Part print with two shaded views. Sizes in mm from the minimum x, y, z corner. A direction names the side the tool comes from. Coordinates: 2 decimals unless noted, no trailing zeros. Loops run counter-clockwise (first coordinate to the right, second up) from the corner with the lowest first, then second, coordinate; pieces in that order, holes last.
Item 1: Cut at C-C (y = 7). List the corners of the cut face in (x, z).
Item 2: Cut at B-B (z = 50). List the corners of the cut face in (x, y), and give its area (3 significant figures).
Item 3: Drill centre lines: line 1 along Z through (x, y) = (31, 47); line 2 along Y through (x, z) = (15, 33); line 3 along Z through (x, y) = (22.5, 21). Where is each one in solid material? Low to high.
Item 4: 3-axis set-ups, long thin cutter, end or side, ignore diameter. For the marked faces 1, 2 and 3: which of +Z, -Z, +X, -X, +Y, -Y reach the whole face in a straight line?
Item 5: Mould opens along X. For the marked faces 4, 5 and 6 say: released by +X, released by -X, zero draft, split by the parting line, or undercut.
Item 6: Flat gauge pins, fed straight in: pin 1 (14 mm diameter, centred on x = 24, z = 4, fed in from -Y); pin 2 (2 mm diameter, centred on x = 20.5, y = 37, fed in from +Z); pin 3 (12 mm diameter, centred on y = 38.5, z = 37.5, fed in from +X); pin 4 (2.5 mm diameter, centred on y = 3.5, z = 9.5, fed in from -X) (1 decimal). Where does each tip first touch, or does it go through?
Item 7: Cut at A-A (x = 31.75). List the corners of the cut face in (y, z), and give its area (3 significant figures).
Item 8: Cut at D-D (y = 15). List the corners of the cut face in (x, z).
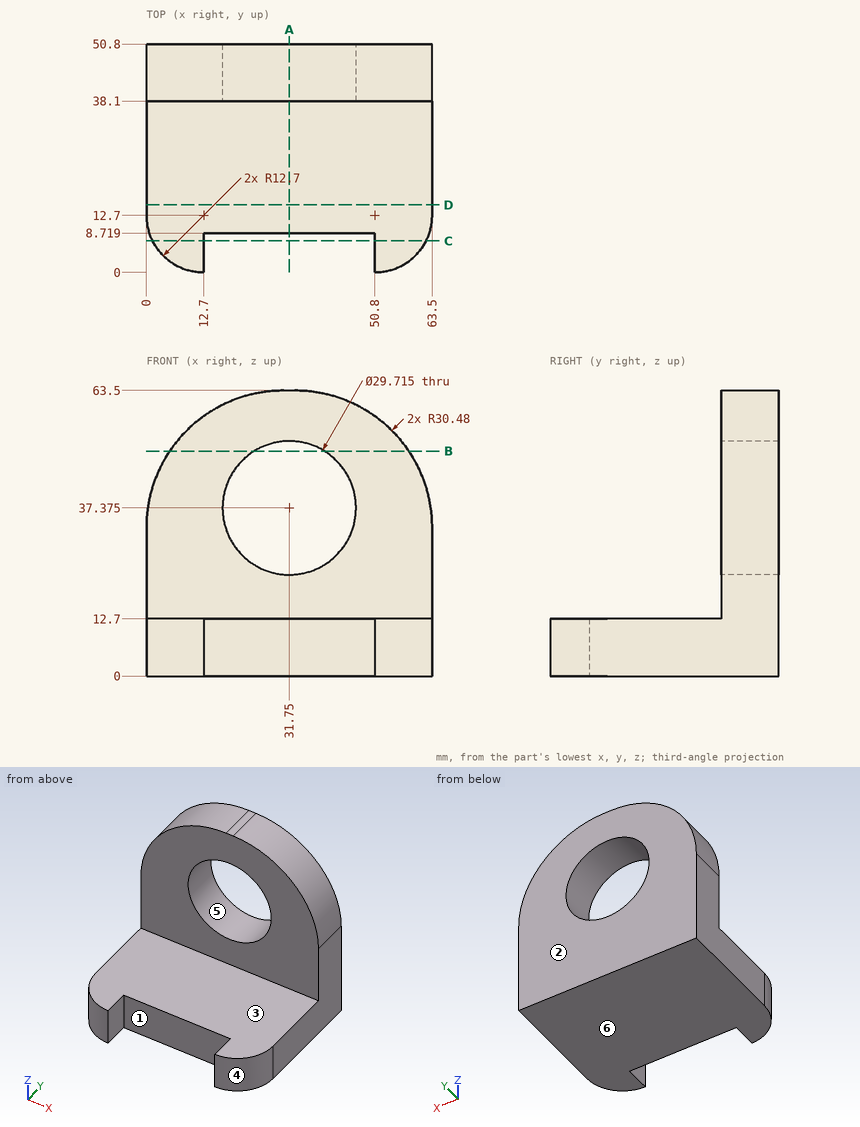
Filled sheet:
1. outline: (1.35, 0) - (12.7, 0) - (12.7, 12.7) - (1.35, 12.7) - close; (50.8, 0) - (62.15, 0) - (62.15, 12.7) - (50.8, 12.7) - close
2. outline: (5.17, 38.1) - (23.92, 38.1) - (23.92, 50.8) - (5.17, 50.8) - close; (39.58, 38.1) - (58.33, 38.1) - (58.33, 50.8) - (39.58, 50.8) - close
2. area: 476 mm2
3. line 1: z = 0 to 22.54, 52.21 to 63.5
3. line 2: y = 38.1 to 50.8
3. line 3: z = 0 to 12.7
4. face 1: +Z, -Z, -Y
4. face 2: +Z, -Z, +X, -X, +Y
4. face 3: +Z, +X, -X, -Y
5. face 4: released by +X
5. face 5: undercut
5. face 6: zero draft
6. pin 1: stops at y = 8.72
6. pin 2: stops at z = 12.7
6. pin 3: stops at x = 63.5
6. pin 4: stops at x = 2.8
7. outline: (8.72, 0) - (50.8, 0) - (50.8, 22.52) - (38.1, 22.52) - (38.1, 12.7) - (8.72, 12.7) - close; (38.1, 52.23) - (50.8, 52.23) - (50.8, 63.5) - (38.1, 63.5) - close
7. area: 802 mm2
8. outline: (0, 0) - (63.5, 0) - (63.5, 12.7) - (0, 12.7) - close
